The model under review builds one solid part; all positions refer to its coordinate system, in mm. Round coordinates to 2 decimals unless told otherwise and drop trailing zeros. Write each loop counter-clockwise with the first axis right and the second up, starting at its lowest first coordinate (ties: lowest second). Pieces come first, ordered by that corner, then holes. Notation, with made-up numbers: (-2, 23) -> (41, 23) arc R19 ccw to (41, 56) -> close; hole circle Ø10 at (8.5, 27). An arc over 180 degrees is marked (long way). Return JSON: item names as keys, results as strings. Group by question number.
1. Take a section at B-B, the plane x = 63. Write out the cut boundary in (y, z).
2. Take a section at A-A, the plane z = 1.8. Write out the cut boundary in (x, y), then the cut area to 3 significant figures.
3. Clearance check with flat-ended pins moving along their axes: P1, Ø1, axis at y = -14.5, z = 2, coming from the -X side; P2, Ø1, axis at x = 57.5, z = 2, coming from the -Y side. State where each tip first meets the part, or that it passes through.
4. Take a section at C-C, the plane y = -21.75. Write out the cut boundary in (x, z), then the cut area to 3 significant figures.
5. For line 1 along X through (y, z) = (-13.75, 1.8); line 2 along Y through (x, z) = (-0.5, 1.55); line 3 along Y through (x, z) = (56.5, 1.85), list the stretches that pass through material, from the lowest coordinate up. Write a range as from..to.
from build123d import *

# Parameters (mm, degrees)
BOSS_EXTRUDE1_DEPTH = 3
FILLET1_R           = 3


with BuildPart() as part:
    # Sketch1 → Boss-Extrude1 (new body)
    with BuildSketch(Plane.XY):
        with BuildLine():
            Line((0, 0), (40, 0))
            Line((40, 0), (66, -5.5))
            ThreePointArc((66, -5.5), (73, -12.5), (66, -19.5))
            Line((66, -19.5), (40, -25))
            Line((40, -25), (0, -25))
            Line((0, -25), (-26, -19.5))
            ThreePointArc((-26, -19.5), (-33, -12.5), (-26, -5.5))
            Line((-26, -5.5), (0, 0))
        make_face()
    extrude(amount=BOSS_EXTRUDE1_DEPTH)

    # Fillet1
    fillet1_edges = [part.edges().sort_by_distance(p)[0] for p in [
        (0, 0, 1.5),
        (40, 0, 1.5),
        (66, -5.5, 1.5),
        (66, -19.5, 1.5),
        (40, -25, 1.5),
        (0, -25, 1.5),
        (-26, -19.5, 1.5),
        (-26, -5.5, 1.5),
    ]]
    fillet(fillet1_edges, radius=FILLET1_R)


solid = part.part
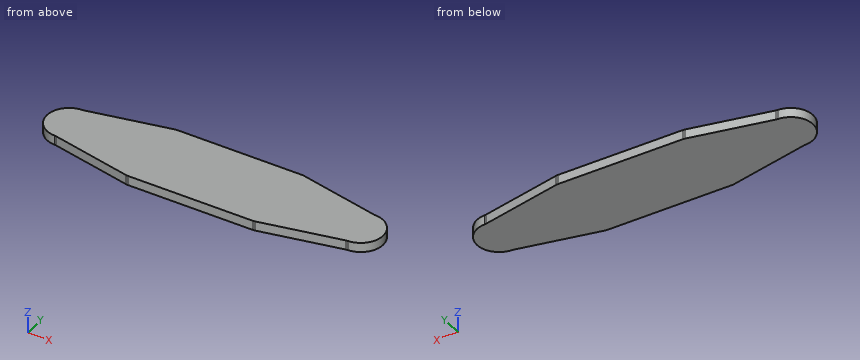
Output:
{
 "1": {"outline": "(-20.13, 0) -> (-4.87, 0) -> (-4.87, 3) -> (-20.13, 3) -> close"},
 "2": {"outline": "(-26.24, -19.5) arc R3 cw to (-25.72, -19.56) -> (-0.31, -24.94) arc R3 ccw to (0.31, -25) -> (39.69, -25) arc R3 ccw to (40.31, -24.94) -> (65.72, -19.56) arc R3 cw to (66.24, -19.5) arc R7 ccw to (66.24, -5.5) arc R3 cw to (65.72, -5.44) -> (40.31, -0.06) arc R3 ccw to (39.69, 0) -> (0.31, 0) arc R3 ccw to (-0.31, -0.06) -> (-25.72, -5.44) arc R3 cw to (-26.24, -5.5) arc R7 ccw to start", "area": "2,170 mm^2"},
 "3": {"P1": "stops at x = -32.84", "P2": "stops at y = -21.4"},
 "4": {"outline": "(-15.36, 0) -> (55.36, 0) -> (55.36, 3) -> (-15.36, 3) -> close", "area": "212 mm^2"},
 "5": {"line 1": "x = -32.89..72.89", "line 2": "y = -24.89..-0.11", "line 3": "y = -21.51..-3.49"}
}
